Source: CAD feature listing. Evaluate the final solid. Frame: model axes, mm. A direction names the side the tool comes from. Round coordinates to 2 decimals unless told otherwise and drop trailing zeros. Write each loop counter-clockwise with the first axis right and the second up, starting at its lowest first coordinate (ties: lowest second). Pieces come first, ordered by that corner, then holes. Notation, with made-up numbers: M -15.75,73 L 16.25,73 A24 cw 16.25,99 Z; hole C 16.5,32 d4. An arc over 180 degrees is marked long. Use a Markdown table: item, result.
```python
from build123d import *

# Parameters (mm, degrees)
SKETCH_1_W          = 25
SKETCH_1_H          = 43.91
EXTRUDE_1_DEPTH     = 7
CUT_EXTRUDE_1_DEPTH = 65
SKETCH_3_R          = 2
CUT_EXTRUDE_2_DEPTH = 65
SKETCH_4_W          = 25
SKETCH_4_H          = 7
EXTRUDE_2_DEPTH     = 10
SKETCH_5_R          = 1.7
EXTRUDE_3_DEPTH     = 25
FILLET_1_R          = 5


with BuildPart() as part:
    # Эскиз1 → Бобышка-Вытянуть1 (new body)
    with BuildSketch(Plane(origin=(0, 0, 0), x_dir=(1, 0, 0), z_dir=(0, 1, 0))):
        with Locations((1252.085571953, -1610.16757215)):
            Rectangle(SKETCH_1_W, SKETCH_1_H)
    extrude(amount=EXTRUDE_1_DEPTH)

    # Эскиз2 → Вырез-Вытянуть1 (cut)
    with BuildSketch(Plane(origin=(1264.585571953, 0, 0), x_dir=(0, 0, -1), z_dir=(1, 0, 0))):
        Polygon((-1594.231269333, 0), (-1599.613127302, 7), (-1588.127511269, 9.94842477), (-1585.312996238, -1.015544634), align=None)
    extrude(amount=-CUT_EXTRUDE_1_DEPTH, mode=Mode.SUBTRACT)

    # Эскиз3 → Вырез-Вытянуть2 (cut)
    with BuildSketch(Plane(origin=(0, 7, 0), x_dir=(1, 0, 0), z_dir=(0, 1, 0))):
        with Locations((1259.585571953, -1602.231269333)):
            Circle(SKETCH_3_R)
        with Locations((1259.585571953, -1625.231269333)):
            Circle(SKETCH_3_R)
        with Locations((1244.585571953, -1602.231269333)):
            Circle(SKETCH_3_R)
        with Locations((1244.585571953, -1625.231269333)):
            Circle(SKETCH_3_R)
    extrude(amount=-CUT_EXTRUDE_2_DEPTH, mode=Mode.SUBTRACT)

    # Эскиз4 → Бобышка-Вытянуть2 (add)
    with BuildSketch(Plane.XY.offset(1632.12257215)):
        with Locations((1252.085571953, 3.5)):
            Rectangle(SKETCH_4_W, SKETCH_4_H)
    extrude(amount=EXTRUDE_2_DEPTH)

    # Эскиз5 → Бобышка-Вытянуть3 (add)
    with BuildSketch(Plane(origin=(1264.585571953, 0, 0), x_dir=(0, 0, -1), z_dir=(1, 0, 0))):
        with BuildLine():
            Line((-1645.661846077, -13.594616806), (-1639.32257215, 0))
            Line((-1639.32257215, 0), (-1642.12257215, 7))
            Line((-1642.12257215, 7), (-1647.092197733, 7))
            Line((-1647.092197733, 7), (-1654.724923947, -9.368434188))
            ThreePointArc((-1654.724923947, -9.368434188), (-1652.30647632, -16.013064432), (-1645.661846077, -13.594616806))
        make_face()
        with Locations((-1650.193385012, -11.481525497)):
            Circle(SKETCH_5_R, mode=Mode.SUBTRACT)
    extrude(amount=-EXTRUDE_3_DEPTH)

    # Скругление1
    fillet_1_edges = [part.edges().sort_by_distance(p)[0] for p in [
        (1252.085571953, 7, 1647.092197733),
    ]]
    fillet(fillet_1_edges, radius=FILLET_1_R)


solid = part.part
```
Q1. Line query: L1, parallel to Y at x = 1242.75, z = 1611.5; L2, parallel to Z at x = 1262, y = -12.75; L3, parallel to X at y = 2.5, z = 1602.5. Output: solid intervals per line, ascending.
Results are:
| item | result |
|---|---|
| L1 | 0 to 7 |
| L2 | 1645.27 to 1649.06, 1651.33 to 1655.03 |
| L3 | 1239.59 to 1242.6, 1246.57 to 1257.6, 1261.57 to 1264.59 |
Q2. First-contact query: pin 1 Ø12 at (x, z) = (1250.5, 1611.5) entering from -Y; pin 2 Ø2 at (x, y) = (1255, -3.5) entering from -Z; pin 3 Ø5 at (x, y) = (1256, 3.5) entering from -Z; pin 4 Ø4.5 at (x, z) = (1259.59, 1625.23) entering from +Y. Flat tips, straight axial feed; report the tip coordinate or a pass-through.
Results are:
| item | result |
|---|---|
| pin 1 | y = 0 |
| pin 2 | z = 1640.49 |
| pin 3 | z = 1595 |
| pin 4 | y = 7 |
Q3. Section D-D on y = 1.25. Return loops of the section in (x, z).
Results are:
| item | result |
|---|---|
| outline | M 1239.59,1595.19 L 1264.59,1595.19 L 1264.59,1649.77 L 1239.59,1649.77 Z; hole C 1244.59,1602.23 d4; hole C 1244.59,1625.23 d4; hole C 1259.59,1602.23 d4; hole C 1259.59,1625.23 d4 |
Q4. Reachability of faces 1 (the cylindrical face through (1251.911, 6.195, 1646.627)), 2 (the flat face through (1252, 0, 1616)) from +Z, -Z, +X, -X, +Y, -Y: full face, straight path, thin tool, end or side. Return the list, or none.
Results are:
| item | result |
|---|---|
| face 1 | +Z, +X, -X, +Y |
| face 2 | -Z, +X, -X, -Y |
Q5. Section C-C on z = 1601. Return loops of the section in (x, y), plus the area to 3 significant figures.
Results are:
| item | result |
|---|---|
| outline | M 1239.59,0 L 1243.01,0 L 1243.01,7 L 1239.59,7 Z; M 1246.16,0 L 1258.01,0 L 1258.01,7 L 1246.16,7 Z; M 1261.16,0 L 1264.59,0 L 1264.59,7 L 1261.16,7 Z |
| area | 131 mm^2 |
Q6. Section B-B on y = -10.5. Return loops of the section in (x, z), plus the area to 3 significant figures.
Results are:
| item | result |
|---|---|
| outline | M 1239.59,1644.22 L 1264.59,1644.22 L 1264.59,1648.81 L 1239.59,1648.81 Z; M 1239.59,1651.58 L 1264.59,1651.58 L 1264.59,1655.1 L 1239.59,1655.1 Z |
| area | 203 mm^2 |
Q7. Section A-A on x = 1245.5. Return loops of the section in (y, z), plus the area to 3 significant figures.
Results are:
| item | result |
|---|---|
| outline | M -13.59,1645.66 L 0,1639.32 L 0,1627.01 L 7,1627.01 L 7,1643.91 A5 ccw 4.11,1648.44 L -9.37,1654.72 A5 ccw Z; M 0,1594.23 L 7,1599.61 L 7,1600.45 L 0,1600.45 Z; M 0,1604.01 L 7,1604.01 L 7,1623.45 L 0,1623.45 Z; hole C -11.48,1650.19 d3.4 |
| area | 468 mm^2 |
Q8. Mould query, pull axis Z, two halves, no side actions, for faces 3 (the flat face through (1252.261, 3.451, 1596.885)), 4 (the flat face through (1252, 7, 1621)), 5 (the cylindrical face through (1259.325, 3.549, 1623.248)), 6 (the flat face through (1252.261, -2.533, 1651.538)). Classes: +Z half, -Z half, draft (parallel to the pull), parting line (faces both ways), or undercut.
Results are:
| item | result |
|---|---|
| face 3 | -Z half |
| face 4 | draft |
| face 5 | undercut |
| face 6 | +Z half |
